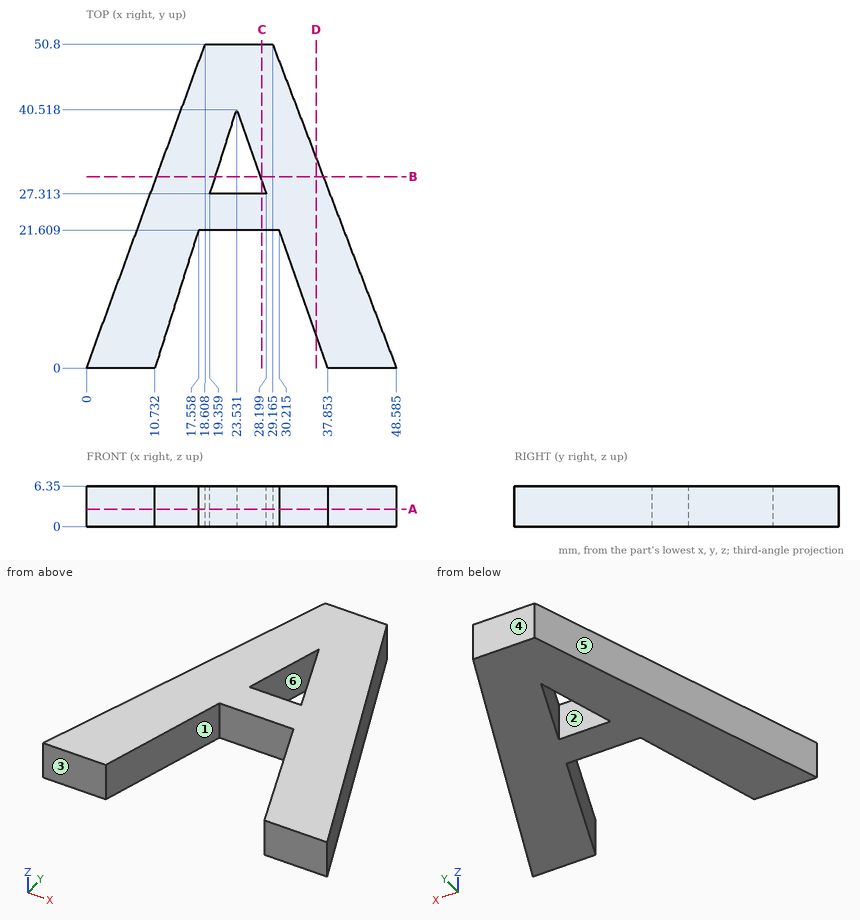
Answer from the drawing. Dimensions are ordinates in mm from the lowest x, y and z of the part. A direction names the side the tool comes from. Round coordinates to 2 decimals unless told otherwise and drop trailing zeros. Loops run counter-clockwise (first coordinate to the right, second up) from the corner with the lowest first, then second, coordinate; pieces in that order, holes last.
Q1. Section A-A on z = 2.75 is taken. Write down the section's boundary in (x, y) (1 decimal), and give its area (3 significant figures).
Q2. Section B-B on y = 30 is taken. Write down the section's boundary in (x, z), and give its area (3 significant figures).
Q3. Section C-C on x = 27.5 is taken. Write down the section's boundary in (y, z).
Q4. Consider probe 1 along X at (y, z) = (29, 1); probe 2 along X at (y, z) = (18, 2) (1 decimal); probe 3 along X at (y, z) = (22.5, 5.5) (1 decimal). Determine where each line is inside the solid, lowest interval first.
Q5. Which of the six approach directions +Z, -Z, +X, -X, +Y, -Y give full straight-line access (tool end or side, diameter ignored) to the marked faces 1, 2 and 3?
Q6. Section D-D on x = 36 is taken. Write down the section's boundary in (y, z).
Q7. Determine the mould class of the marked faces 4, 5 and 6 for opening direction X: released by +X, released by -X, zero draft, split by the parting line, or undercut.
Q8. This flat-tipped pin is pushed along its axis until it touches: pin 1 (2 mm diameter, centred on x = 6.5, y = 26, fed in from +Z). Where does it stop, or does it pass through?
Output:
1. outline: (0, 0) - (10.7, 0) - (17.6, 21.6) - (30.2, 21.6) - (37.9, 0) - (48.6, 0) - (29.2, 50.8) - (18.6, 50.8) - close; hole (19.4, 27.3) - (28.2, 27.3) - (23.5, 40.5) - close
1. area: 1,010 mm2
2. outline: (10.99, 0) - (20.21, 0) - (20.21, 6.35) - (10.99, 6.35) - close; (27.25, 0) - (37.12, 0) - (37.12, 6.35) - (27.25, 6.35) - close
2. area: 121 mm2
3. outline: (21.61, 0) - (27.31, 0) - (27.31, 6.35) - (21.61, 6.35) - close; (29.29, 0) - (50.8, 0) - (50.8, 6.35) - (29.29, 6.35) - close
4. probe 1: x = 10.62 to 19.89, 27.6 to 37.5
4. probe 2: x = 6.6 to 16.4, 31.5 to 41.7
4. probe 3: x = 8.2 to 40
5. face 1: +Z, -Z, -Y
5. face 2: +Z, -Z
5. face 3: +Z, -Z, +X, -X, -Y
6. outline: (5.24, 0) - (32.92, 0) - (32.92, 6.35) - (5.24, 6.35) - close
7. face 4: zero draft
7. face 5: released by -X
7. face 6: undercut
8. pin 1: passes through
